from build123d import *

# Parameters (mm, degrees)
SKETCH1_W           = 14
SKETCH1_H           = 41.5
SKETCH1_R           = 2.1
SKETCH1_W_2         = 1
SKETCH1_H_2         = 5
BOSS_EXTRUDE3_DEPTH = 15.3
SKETCH2_W           = 10.3
SKETCH2_H           = 17
SKETCH2_H_2         = 21.5
CUT_EXTRUDE1_DEPTH  = 21


with BuildPart() as part:
    # Sketch1 → Boss-Extrude3 (new body)
    # profile 1 of 3: a face of its own
    with BuildSketch(Plane.XY):
        with Locations((7, 20.75)):
            Rectangle(SKETCH1_W, SKETCH1_H)
        with Locations((3, 10)):
            Circle(SKETCH1_R, mode=Mode.SUBTRACT)
        with Locations((11, 10)):
            Circle(SKETCH1_R, mode=Mode.SUBTRACT)
        Polygon((3.3, 38.5), (4.3, 38.5), (9.7, 38.5), (10.7, 38.5), (11, 38.5), (11, 33.5), (10.7, 33.5), (9.7, 33.5), (4.3, 33.5), (3.3, 33.5), (3, 33.5), (3, 38.5), align=None, mode=Mode.SUBTRACT)
    # profile 2 of 3: a face of its own
    with BuildSketch(Plane.XY):
        with Locations((3.8, 36)):
            Rectangle(SKETCH1_W_2, SKETCH1_H_2)
    # profile 3 of 3: a face of its own
    with BuildSketch(Plane.XY):
        with Locations((10.2, 36)):
            Rectangle(SKETCH1_W_2, SKETCH1_H_2)
    extrude(amount=BOSS_EXTRUDE3_DEPTH)

    # Sketch2 → Cut-Extrude1 (cut)
    with BuildSketch(Plane.ZY):
        with Locations((5.15, 8.5)):
            Rectangle(SKETCH2_W, SKETCH2_H)
        with Locations((10.15, 30.75)):
            Rectangle(SKETCH2_W, SKETCH2_H_2)
    extrude(amount=-CUT_EXTRUDE1_DEPTH, mode=Mode.SUBTRACT)


solid = part.part
Can you work these out from the model? Positions are in its coordinate system, mm. A direction names the side the tool comes from. Coordinates: 2 decimals unless noted, no trailing zeros. Loops run counter-clockwise (first coordinate to the right, second up) from the corner with the lowest first, then second, coordinate; pieces in that order, holes last. Notation, with made-up numbers: (1, 58) - (55, 58) arc R29 ccw to (55, 79) - close; hole circle Ø3 at (53.5, 30.25). An arc over 180 degrees is marked (long way). Put each result on its own line as item: value. Start each with the question number.
Item 1: If we mould it in two halves opening along X, with no side actions, what happens to faces 5 (the face through (14, 19, 7)), 6 (the face through (7, 0, 13)), 7 (the face through (7, 38.5, 2)), 8 (the face through (0, 19, 7))? For each: +X half, -X half, draft (parallel to the pull), parting line (faces both ways), or undercut.
Item 2: Suppose I cut it at C-C (y = 34.5). Please give me the cut outline in (x, z), and give its area (3 significant figures).
Item 3: Which directions (+Z, -Z, +X, -X, +Y, -Y) give clear straight access to the entire face, cutting with the end or side of a thin tool? Please do faces 1 (the face through (7, 8, 10.3)), 2 (the face through (7, 31, 5)), 3 (the face through (7, 10, 15.3)), 4 (the face through (3, 36, 2)).
Item 4: Suppose I cut it at D-D (z = 3.25). Please give me the cut outline in (x, y), and give its area (3 significant figures).
Item 5: Suppose I cut it at A-A (y = 10). Please give me the cut outline in (x, z).
Item 6: If I drill on line 1 along X through (y, z) = (10, 11.6); line 2 along Y through (x, z) = (7.5, 4.25); line 3 along Y through (x, z) = (3, 13.15), over which ranges is the centre line in solid material (lowest first)?
Item 7: For pin 1 (3 mm diameter, centred on x = 2, z = 2.5, fed in from -Y); pin 2 (4 mm diameter, centred on x = 9, y = 36, fed in from +Z); pin 3 (5 mm diameter, centred on x = 11, y = 10, fed in from -Z), each with a flat end and sliding along its axis, tell me the tip position at first contact or that it passes through.
Item 8: Suppose I cut it at B-B (x = 8.25). Please give me the cut outline in (y, z), and give its area (3 significant figures).
Here are the results:
1. face 5: +X half
1. face 6: draft
1. face 7: undercut
1. face 8: -X half
2. outline: (0, 0) - (3, 0) - (3, 5) - (0, 5) - close; (3.3, 0) - (4.3, 0) - (4.3, 5) - (3.3, 5) - close; (9.7, 0) - (10.7, 0) - (10.7, 5) - (9.7, 5) - close; (11, 0) - (14, 0) - (14, 5) - (11, 5) - close
2. area: 40.0 mm²
3. face 1: -Z, +X, -X, -Y
3. face 2: +Z, +X, -X, +Y
3. face 3: +Z, +X, -X, +Y, -Y
3. face 4: +Z, -Z
4. outline: (0, 17) - (14, 17) - (14, 41.5) - (0, 41.5) - close; hole (3, 33.5) - (3.3, 33.5) - (3.3, 38.5) - (3, 38.5) - close; hole (4.3, 33.5) - (9.7, 33.5) - (9.7, 38.5) - (4.3, 38.5) - close; hole (10.7, 33.5) - (11, 33.5) - (11, 38.5) - (10.7, 38.5) - close
4. area: 313 mm²
5. outline: (0, 10.3) - (0.9, 10.3) - (0.9, 15.3) - (0, 15.3) - close; (5.1, 10.3) - (8.9, 10.3) - (8.9, 15.3) - (5.1, 15.3) - close; (13.1, 10.3) - (14, 10.3) - (14, 15.3) - (13.1, 15.3) - close
6. line 1: 0 to 0.9, 5.1 to 8.9, 13.1 to 14
6. line 2: 17 to 33.5, 38.5 to 41.5
6. line 3: 0 to 7.9, 12.1 to 20
7. pin 1: y = 17
7. pin 2: z = 5
7. pin 3: z = 10.3
8. outline: (0, 10.3) - (17, 10.3) - (17, 0) - (33.5, 0) - (33.5, 5) - (20, 5) - (20, 15.3) - (0, 15.3) - close; (38.5, 0) - (41.5, 0) - (41.5, 5) - (38.5, 5) - close
8. area: 213 mm²
